from build123d import *

# Parameters (mm, degrees)
EXTRUDE_1_DEPTH     = 30
CUT_EXTRUDE_1_REACH = 63.952
SKETCH_4_R          = 2
CUT_EXTRUDE_2_REACH = 62.407
SKETCH_5_R          = 2.5
SKETCH_5_R_2        = 1.5


with BuildPart() as part:
    # 草图2 → 凸台-拉伸1 (new body)
    with BuildSketch(Plane(origin=(0, 0, 0), x_dir=(1, 0, 0), z_dir=(0, 1, 0))):
        Polygon((0, 0), (43, 0), (43, 3), (3, 3), (3, 33), (0, 33), align=None)
    extrude(amount=EXTRUDE_1_DEPTH)

    # 草图4 → 切除-拉伸1 (cut, up to next)
    with BuildSketch(Plane.ZY, mode=Mode.PRIVATE) as cut_extrude_1_sk1:
        with Locations((-18, 7.5)):
            Circle(SKETCH_4_R)
    cut_extrude_1_tool1 = extrude(cut_extrude_1_sk1.sketch, amount=-CUT_EXTRUDE_1_REACH, mode=Mode.PRIVATE) & part.part
    # 草图4 → 切除-拉伸1 (cut, up to next)
    with BuildSketch(Plane.ZY, mode=Mode.PRIVATE) as cut_extrude_1_sk2:
        with Locations((-18, 22.5)):
            Circle(SKETCH_4_R)
    cut_extrude_1_tool2 = extrude(cut_extrude_1_sk2.sketch, amount=-CUT_EXTRUDE_1_REACH, mode=Mode.PRIVATE) & part.part
    add(cut_extrude_1_tool1.solids().sort_by_distance((0, 7.5, -18))[0], mode=Mode.SUBTRACT)
    add(cut_extrude_1_tool2.solids().sort_by_distance((0, 22.5, -18))[0], mode=Mode.SUBTRACT)

    # 草图5 → 切除-拉伸2 (cut, up to next)
    with BuildSketch(Plane(origin=(0, 0, -3), x_dir=(-1, 0, 0), z_dir=(0, 0, -1)), mode=Mode.PRIVATE) as cut_extrude_2_sk1:
        with Locations((-15, 15)):
            Circle(SKETCH_5_R)
    cut_extrude_2_tool1 = extrude(cut_extrude_2_sk1.sketch, amount=-CUT_EXTRUDE_2_REACH, mode=Mode.PRIVATE) & part.part
    # 草图5 → 切除-拉伸2 (cut, up to next)
    with BuildSketch(Plane(origin=(0, 0, -3), x_dir=(-1, 0, 0), z_dir=(0, 0, -1)), mode=Mode.PRIVATE) as cut_extrude_2_sk2:
        with Locations((-20.656854249, 9.343145751)):
            Circle(SKETCH_5_R_2)
    cut_extrude_2_tool2 = extrude(cut_extrude_2_sk2.sketch, amount=-CUT_EXTRUDE_2_REACH, mode=Mode.PRIVATE) & part.part
    # 草图5 → 切除-拉伸2 (cut, up to next)
    with BuildSketch(Plane(origin=(0, 0, -3), x_dir=(-1, 0, 0), z_dir=(0, 0, -1)), mode=Mode.PRIVATE) as cut_extrude_2_sk3:
        with Locations((-9.343145751, 9.343145751)):
            Circle(SKETCH_5_R_2)
    cut_extrude_2_tool3 = extrude(cut_extrude_2_sk3.sketch, amount=-CUT_EXTRUDE_2_REACH, mode=Mode.PRIVATE) & part.part
    # 草图5 → 切除-拉伸2 (cut, up to next)
    with BuildSketch(Plane(origin=(0, 0, -3), x_dir=(-1, 0, 0), z_dir=(0, 0, -1)), mode=Mode.PRIVATE) as cut_extrude_2_sk4:
        with Locations((-20.656854249, 20.656854249)):
            Circle(SKETCH_5_R_2)
    cut_extrude_2_tool4 = extrude(cut_extrude_2_sk4.sketch, amount=-CUT_EXTRUDE_2_REACH, mode=Mode.PRIVATE) & part.part
    # 草图5 → 切除-拉伸2 (cut, up to next)
    with BuildSketch(Plane(origin=(0, 0, -3), x_dir=(-1, 0, 0), z_dir=(0, 0, -1)), mode=Mode.PRIVATE) as cut_extrude_2_sk5:
        with Locations((-9.343145751, 20.656854249)):
            Circle(SKETCH_5_R_2)
    cut_extrude_2_tool5 = extrude(cut_extrude_2_sk5.sketch, amount=-CUT_EXTRUDE_2_REACH, mode=Mode.PRIVATE) & part.part
    add(cut_extrude_2_tool1.solids().sort_by_distance((15, 15, -3))[0], mode=Mode.SUBTRACT)
    add(cut_extrude_2_tool2.solids().sort_by_distance((20.656854, 9.343146, -3))[0], mode=Mode.SUBTRACT)
    add(cut_extrude_2_tool3.solids().sort_by_distance((9.343146, 9.343146, -3))[0], mode=Mode.SUBTRACT)
    add(cut_extrude_2_tool4.solids().sort_by_distance((20.656854, 20.656854, -3))[0], mode=Mode.SUBTRACT)
    add(cut_extrude_2_tool5.solids().sort_by_distance((9.343146, 20.656854, -3))[0], mode=Mode.SUBTRACT)


solid = part.part
Can you work these out from the model? Positions are in its coordinate system, mm. A direction names the side the tool comes from. Round coordinates to 2 decimals unless told otherwise and drop trailing zeros. Write each loop counter-clockwise with the first axis right and the second up, starting at its lowest first coordinate (ties: lowest second). Pieces come first, ordered by that corner, then holes. Notation, with made-up numbers: (-29, 87.5) - (21, 87.5) arc R23 cw to (21, 118.5) - close; hole circle Ø2 at (9, 14.25). An arc over 180 degrees is marked (long way). Write each question's results on one line, items separated by ' | '. Start each with the question number.
1) For pin 1 Ø2 at (y, z) = (21, -10) entering from +X, with a flat end and sliding along its axis, tell me the tip position at first contact or that it passes through.
2) Which directions (+Z, -Z, +X, -X, +Y, -Y) give clear straight access to the entire face, cutting with the end or side of a thin tool? Please do faces 1 (the flat face through (3, 15, -18)), 2 (the flat face through (2, 15, -33)).
3) We'd pull the mould along Z, two halves only. Please class faces 3 (the flat face through (23, 15, -3)), 4 (the flat face through (21, 15, 0)), 5 (the flat face through (12, 30, -2)), 6 (the cylindrical face through (1.479, 8.852, -19.474)): released by +Z, released by -Z, zero draft, split by the parting line, or undercut.
4) Suppose I cut it at B-B (x = 15). List the corners of the cut face in (y, z) for me.
5) Suppose I cut it at D-D (y = 25.5). List the corners of the cut face in (x, z) for me.
6) Suppose I cut it at C-C (z = -18). List the corners of the cut face in (x, y) for me.
7) Suppose I cut it at A-A (y = 15). List the corners of the cut face in (x, z) for me.
8) Please list where these lines run through material, in increasing order: line 1 (Y direction, x = 0.75, z = -18); line 2 (X direction, y = 13.75, z = -14.5); line 3 (Z direction, x = 18, y = 28.5).
Here are the results:
1) pin 1: stops at x = 3
2) face 1: -Z, +X, +Y, -Y | face 2: -Z, +X, -X, +Y, -Y
3) face 3: released by -Z | face 4: released by +Z | face 5: zero draft | face 6: undercut
4) outline: (0, -3) - (12.5, -3) - (12.5, 0) - (0, 0) - close; (17.5, -3) - (30, -3) - (30, 0) - (17.5, 0) - close
5) outline: (0, -33) - (3, -33) - (3, -3) - (43, -3) - (43, 0) - (0, 0) - close
6) outline: (0, 0) - (3, 0) - (3, 5.5) - (0, 5.5) - close; (0, 9.5) - (3, 9.5) - (3, 20.5) - (0, 20.5) - close; (0, 24.5) - (3, 24.5) - (3, 30) - (0, 30) - close
7) outline: (0, -33) - (3, -33) - (3, -3) - (12.5, -3) - (12.5, 0) - (0, 0) - close; (17.5, -3) - (43, -3) - (43, 0) - (17.5, 0) - close
8) line 1: y = 0 to 5.5, 9.5 to 20.5, 24.5 to 30 | line 2: x = 0 to 3 | line 3: z = -3 to 0
